For this review, take the finished solid that the model builds, in its own axes (mm). A direction names the side the tool comes from. Give positions to 0.01 mm unless a question says otherwise; leave off trailing zeros. Loops run counter-clockwise (first coordinate to the right, second up) from the corner with the lowest first, then second, coordinate; pieces in that order, holes last. Notation, with made-up numbers: (79, 79.5) - (107, 79.5) arc R3 cw to (107, 83.5) - close; hole circle Ø8 at (68, 69). An arc over 180 degrees is marked (long way). Answer in a Markdown table with one row per item.
```python
from build123d import *

# Parameters (mm, degrees)
F1_DEPTH = 4
F2_R     = 0.75
F3_DEPTH = 25
F4_R     = 0.75
F5_DEPTH = 25


with BuildPart() as f1:
    # F0 (on Front) → F1 (new body, symmetric)
    with BuildSketch(Plane.XZ):
        Polygon((4, -4), (4, 4), (-4, -4), align=None)
    extrude(amount=F1_DEPTH, both=True)

    # F2 (on Top) → F3 (join)
    with BuildSketch(Plane.XY):
        Circle(F2_R)
    extrude(amount=F3_DEPTH)

    # F4 (on Right) → F5 (join)
    with BuildSketch(Plane.YZ):
        Circle(F4_R)
    extrude(amount=-F5_DEPTH)


solid = f1.part
```
1. Wall thickness on line 1 (X direction, y = 0, z = 14.5); line 2 (Z direction, x = 0, y = -3): over which ranges is each line inside the solid? List them lowest first. Write a range as [from, to].
Values:
| item | result |
|---|---|
| line 1 | x = [-0.75, 0.75] |
| line 2 | z = [-4, 0] |
2. We need section B-B, the plane x = -9. Give the boundary of the cut face in (y, z).
Values:
| item | result |
|---|---|
| outline | circle Ø1.5 at (0, 0) |
3. We need section C-C, the plane z = -1.75. Give the boundary of the cut face in (x, y).
Values:
| item | result |
|---|---|
| outline | (-1.75, -4) - (4, -4) - (4, 4) - (-1.75, 4) - close |
4. For faces 1 (the face through (0, 0, 25)), 2 (the face through (0.715, 0.225, 12.325)), list the 3-axis set-ups (+Z, -Z, +X, -X, +Y, -Y) from which the entire face can be reached by the end or side of a thin tool; tool diameter is ignored.
Values:
| item | result |
|---|---|
| face 1 | +Z, +X, -X, +Y, -Y |
| face 2 | +Z |
5. Clearance check with flat-ended pins moving along their axes: pin 1 (12 mm diameter, centred on x = -1, z = 10.5, fed in from +Y); pin 2 (1 mm diameter, centred on y = 1, z = 18.5, fed in from -X); pin 3 (3 mm diameter, centred on y = 1.5, z = 8.5, fed in from -X). State where each tip first meets the part, or that it passes through.
Values:
| item | result |
|---|---|
| pin 1 | stops at y = 0.75 |
| pin 2 | stops at x = -0.56 |
| pin 3 | stops at x = -0.75 |
6. We need section D-D, the plane y = -1.5. Give the boundary of the cut face in (x, z).
Values:
| item | result |
|---|---|
| outline | (-4, -4) - (4, -4) - (4, 4) - close |
7. Mouldability with a two-part tool opening along X and no side actions: class faces 3 (the face through (-25, 0, 0)), 4 (the face through (4, 0, 0)), 5 (the face through (-12.32, -0.75, 0.03)) as released by +X, released by -X, zero draft, split by the parting line, or undercut.
Values:
| item | result |
|---|---|
| face 3 | released by -X |
| face 4 | released by +X |
| face 5 | zero draft |
